Build history of the part. All positions in model axes, mm. Face numbers are marked on the shaded views. A direction names the side the tool comes from. Round coordinates to 2 decimals unless told otherwise and drop trailing zeros. Order: outer loops, then holes, each group sorted by start corner. A loop starts at its lowest first (then second) coordinate and runs counter-clockwise, first axis right, second up. Notation, with made-up numbers: (-28, 80.5) -> (14, 80.5) arc R28 cw to (14, 107.5) -> close; hole circle Ø4 at (32, 30). An arc over 180 degrees is marked (long way). Use a Markdown table: item, result. Add a question column.
Item 1: 3-axis set-ups, long thin cutter, end or side, ignore diameter. For the marked faces 1 and 2: which of +Z, -Z, +X, -X, +Y, -Y reach the whole face in a straight line?
Item 2: Pin check, flat tips, straight feed: pin 1 (2 mm diameter, centred on y = -6.5, z = 3.5, fed in from -X); pin 2 (2 mm diameter, centred on x = 3.5, z = 3, fed in from -Y); pin 3 (1 mm diameter, centred on x = -1.5, z = 2.5, fed in from -Y). Stop position of each tip, or through.
Item 3: Probe L1, parallel to Y at x = 0, z = 1.8; L2, parallel to X at y = 0, z = 3.6; L3, parallel to Z at x = -8, y = 18. List the from-to ranges inside material, lowest first.
Item 4: Slice it at B-B, the plane y = 33.5. Give the cut face in (x, z).
Item 5: Slice it at D-D, the plane y = 0. Give the cut face in (x, z), plus the area to 3 significant figures.
Item 6: Two-plate mould, pull along Y, no slides. Class the marked faces 3, 4, 5 and 6: released by +Y, released by -Y, zero draft, split by the parting line, or undercut.
Item 7: Slice it at C-C, the plane z = 2.8. Give the cut face in (x, y), plus the area to 3 significant figures.
Item 8: Slice it at A-A, the plane x = 0. Give the cut face in (y, z), plus the area to 3 significant figures.
from build123d import *

# Parameters (mm, degrees)
SKETCH003_R  = 3
PAD001_DEPTH = 1
SKETCH_R     = 3
PAD_DEPTH    = 4


with BuildPart() as bottom_body:
    # Sketch003 → Pad001 (new body)
    with BuildSketch(Plane.XY):
        with BuildLine():
            Line((-17.323639, 4.887895), (-7.982505, 37.994419))
            ThreePointArc((-5.095233, 40.179764), (-6.905763, 39.571831), (-7.982505, 37.994419))
            Line((-5.095233, 40.179764), (6.389044, 40.179764))
            ThreePointArc((9.304202, 37.88818), (8.24306, 39.538286), (6.389044, 40.179764))
            Line((9.304202, 37.88818), (17.323639, 4.887895))
            ThreePointArc((-17.323639, 4.887895), (0, -18), (17.323639, 4.887895))
        make_face()
        with Locations((0, 34.821754)):
            Circle(SKETCH003_R, mode=Mode.SUBTRACT)
    extrude(amount=PAD001_DEPTH)


with BuildPart() as fusion:
    # Sketch → Pad (new body)
    with BuildSketch(Plane.XY):
        with BuildLine():
            Line((-17.323639, 4.887895), (-7.982505, 37.994419))
            ThreePointArc((-5.095233, 40.179764), (-6.905763, 39.571831), (-7.982505, 37.994419))
            Line((-5.095233, 40.179764), (6.389044, 40.179764))
            ThreePointArc((9.304202, 37.88818), (8.24306, 39.538286), (6.389044, 40.179764))
            Line((9.304202, 37.88818), (17.323639, 4.887895))
            ThreePointArc((-17.323639, 4.887895), (0, -18), (17.323639, 4.887895))
        make_face()
        with Locations((0, 34.821754)):
            Circle(SKETCH_R, mode=Mode.SUBTRACT)
        with BuildLine():
            Line((-15.333297, 4.57056), (-8, 29.174304))
            Line((-8, 29.174304), (8, 29.174304))
            Line((8, 29.174304), (15.333297, 4.57056))
            ThreePointArc((-15.333297, 4.57056), (0, -16), (15.333297, 4.57056))
        make_face(mode=Mode.SUBTRACT)
    extrude(amount=PAD_DEPTH)


with BuildPart() as fusion_1:
    # Body placement: moved
    add(fusion.part.moved(Location((0, 0, 1))))

    # Fusion: union bottom body
    add(bottom_body.part)


solid = fusion_1.part
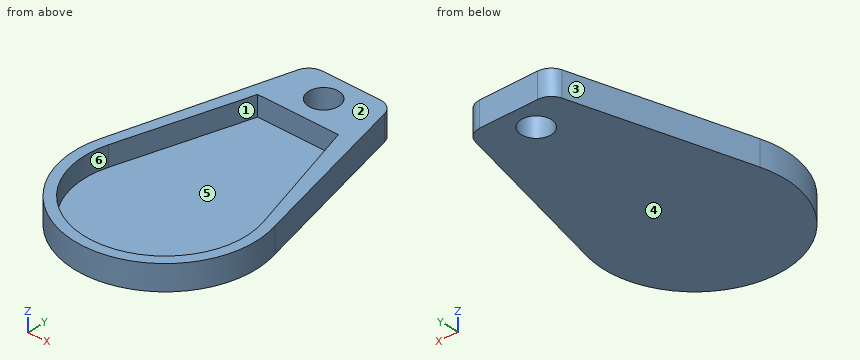
Check sheet entries:
| question | item | result |
|---|---|---|
| 1 | face 1 | +Z |
| 1 | face 2 | +Z, +X, -X, +Y, -Y |
| 2 | pin 1 | x = -17.14 |
| 2 | pin 2 | y = -17.83 |
| 2 | pin 3 | y = -17.97 |
| 3 | L1 | -18 to -16, 29.17 to 31.82, 37.82 to 40.18 |
| 3 | L2 | -18 to -16, 16 to 18 |
| 3 | L3 | 0 to 1 |
| 4 | outline | (-9.25, 0) -> (-2.69, 0) -> (-2.69, 5) -> (-9.25, 5) -> close; (2.69, 0) -> (10.37, 0) -> (10.37, 5) -> (2.69, 5) -> close |
| 5 | outline | (-18, 0) -> (18, 0) -> (18, 5) -> (16, 5) -> (16, 1) -> (-16, 1) -> (-16, 5) -> (-18, 5) -> close |
| 5 | area | 52.0 mm2 |
| 6 | face 3 | released by +Y |
| 6 | face 4 | zero draft |
| 6 | face 5 | undercut |
| 6 | face 6 | undercut |
| 7 | outline | (-17.32, 4.89) arc R18 ccw (long way) to (17.32, 4.89) -> (9.3, 37.89) arc R3 ccw to (6.39, 40.18) -> (-5.1, 40.18) arc R3 ccw to (-7.98, 37.99) -> close; hole (-15.33, 4.57) arc R16 ccw (long way) to (15.33, 4.57) -> (8, 29.17) -> (-8, 29.17) -> close; hole circle Ø6 at (0, 34.82) |
| 7 | area | 428 mm2 |
| 8 | outline | (-18, 0) -> (31.82, 0) -> (31.82, 5) -> (29.17, 5) -> (29.17, 1) -> (-16, 1) -> (-16, 5) -> (-18, 5) -> close; (37.82, 0) -> (40.18, 0) -> (40.18, 5) -> (37.82, 5) -> close |
| 8 | area | 80.2 mm2 |
